Model file for the job. Use its own axes, mm. Round coordinates to 2 decimals unless told otherwise and drop trailing zeros. Loops run counter-clockwise (first coordinate to the right, second up) from the corner with the lowest first, then second, coordinate; pieces in that order, holes last. Notation, with made-up numbers: (-35, 60.5) - (-6, 60.5) arc R13 cw to (-6, 79.5) - close; hole circle Ø5 at (1.25, -1). An arc over 180 degrees is marked (long way). Answer as a JSON object with one key per item and string values.
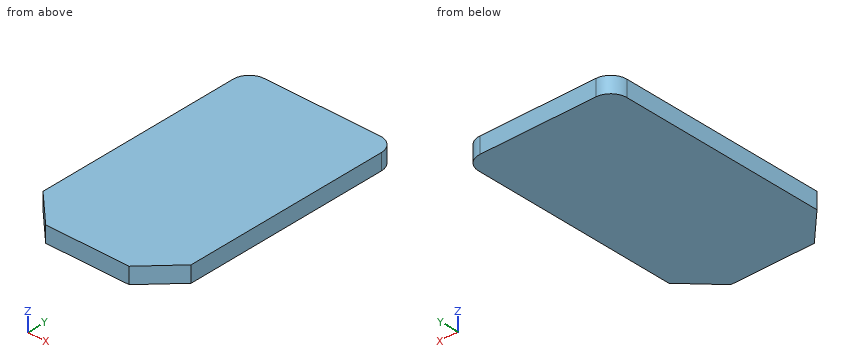
from build123d import *

# Parameters (mm, degrees)
F1_DEPTH = 3


with BuildPart() as f1:
    # F0 (on Top) → F1 (new body)
    with BuildSketch(Plane.XY):
        with BuildLine():
            Line((-46.185345, 45.218922), (-67.685345, 45.218922))
            ThreePointArc((-67.685345, 45.218922), (-69.806666, 44.340243), (-70.685345, 42.218922))
            Line((-70.685345, 42.218922), (-70.685345, 3.718922))
            Line((-70.685345, 3.718922), (-64.685345, -2.281078))
            Line((-64.685345, -2.281078), (-49.185345, -2.281078))
            Line((-49.185345, -2.281078), (-43.185345, 3.718922))
            Line((-43.185345, 3.718922), (-43.185345, 42.218922))
            ThreePointArc((-43.185345, 42.218922), (-44.064025, 44.340243), (-46.185345, 45.218922))
        make_face()
    extrude(amount=F1_DEPTH)


solid = f1.part
1) Drop a flat-ended pin along its axis: P1, Ø8, axis at x = -58, y = 13, coming from the -Z side. Give the stop position or say it passes through.
Values follow:
{"P1": "z = 0"}
2) Slice it at B-B on x = -46.75. List the corners of the cut face in (y, z).
Values follow:
{"outline": "(0.15, 0) - (45.22, 0) - (45.22, 3) - (0.15, 3) - close"}
3) Slice it at A-A on z = 1.75. List the corners of the cut face in (x, y), then the cut area to 3 significant figures.
Values follow:
{"outline": "(-70.69, 3.72) - (-64.69, -2.28) - (-49.19, -2.28) - (-43.19, 3.72) - (-43.19, 42.22) arc R3 ccw to (-46.19, 45.22) - (-67.69, 45.22) arc R3 ccw to (-70.69, 42.22) - close", "area": "1,270 mm²"}
4) Probe probe 1 along X at (y, z) = (0.5, 2.35); probe 2 along Y at (x, z) = (-68.5, 2.7); probe 3 along Y at (x, z) = (-46.5, 2.4). List the from-to ranges inside material, lowest first.
Values follow:
{"probe 1": "-67.47 to -46.4", "probe 2": "1.53 to 45.11", "probe 3": "0.4 to 45.22"}
